Can you work these out from the model? Positions are in its coordinate system, mm. Face numbers are marked on the shaded views. A direction names the side the tool comes from. Round coordinates to 2 decimals unless told otherwise and drop trailing zeros. Loops run counter-clockwise (first coordinate to the right, second up) from the corner with the lowest first, then second, coordinate; pieces in that order, holes last. Notation, with made-up numbers: (1, 40.5) - (58, 40.5) arc R21 cw to (58, 59.5) - close; hole circle Ø4 at (4.5, 21). An arc over 180 degrees is marked (long way). Answer as CSV lines item,"result".
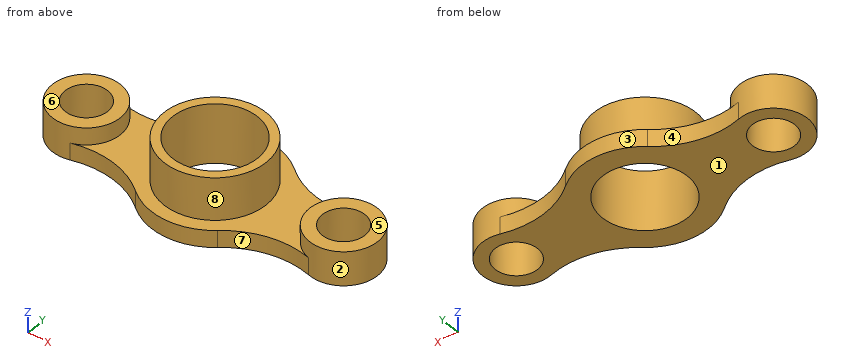
```python
from build123d import *

# Parameters (mm, degrees)
SKETCH2_R           = 60
BOSS_EXTRUDE1_DEPTH = 20
SKETCH2_5_R         = 40
SKETCH2_5_R_2       = 25
BOSS_EXTRUDE4_DEPTH = 40
SKETCH2_6_R         = 60
SKETCH2_6_R_2       = 50
BOSS_EXTRUDE5_DEPTH = 70


with BuildPart() as part:
    # Sketch2 → Boss-Extrude1 (new body)
    with BuildSketch(Plane.XY):
        with BuildLine():
            ThreePointArc((-139.071428571, -38.478127898), (-91.104177178, -36.827906099), (-47.892857143, -57.717191847))
            ThreePointArc((-47.892857143, -57.717191847), (0, -75), (47.892857143, -57.717191847))
            ThreePointArc((47.892857143, -57.717191847), (91.104177178, -36.827906099), (139.071428571, -38.478127898))
            ThreePointArc((139.071428571, -38.478127898), (110, 0), (139.071428571, 38.478127898))
            ThreePointArc((139.071428571, 38.478127898), (91.104177178, 36.827906099), (47.892857143, 57.717191847))
            ThreePointArc((47.892857143, 57.717191847), (0, 75), (-47.892857143, 57.717191847))
            ThreePointArc((-47.892857143, 57.717191847), (-91.104177178, 36.827906099), (-139.071428571, 38.478127898))
            ThreePointArc((-139.071428571, 38.478127898), (-118.084934144, 24.112830017), (-110, 0))
            ThreePointArc((-110, 0), (-118.084934144, -24.112830017), (-139.071428571, -38.478127898))
        make_face()
        Circle(SKETCH2_R, mode=Mode.SUBTRACT)
    extrude(amount=BOSS_EXTRUDE1_DEPTH)

    # Sketch2_5 → Boss-Extrude4 (add)
    # profile 1 of 2: a face of its own
    with BuildSketch(Plane.XY):
        with Locations(Location((-150, 0, 0), (0, 0, 74.144374523))):
            Circle(SKETCH2_5_R)
        with Locations((-150, 0)):
            Circle(SKETCH2_5_R_2, mode=Mode.SUBTRACT)
    # profile 2 of 2: a face of its own
    with BuildSketch(Plane.XY):
        with Locations(Location((150, 0, 0), (0, 0, 105.855625477))):
            Circle(SKETCH2_5_R)
        with Locations((150, 0)):
            Circle(SKETCH2_5_R_2, mode=Mode.SUBTRACT)
    extrude(amount=BOSS_EXTRUDE4_DEPTH)

    # Sketch2_6 → Boss-Extrude5 (add)
    with BuildSketch(Plane.XY):
        Circle(SKETCH2_6_R)
        Circle(SKETCH2_6_R_2, mode=Mode.SUBTRACT)
    extrude(amount=BOSS_EXTRUDE5_DEPTH)


solid = part.part
```
Q1. Imagine slicing it at A-A (x = -150). Write out the boundary of the cut face in (y, z).
Checks:
outline,"(-40, 0) - (-25, 0) - (-25, 40) - (-40, 40) - close; (25, 0) - (40, 0) - (40, 40) - (25, 40) - close"
Q2. We'd pull the mould along X, two halves only. Please class the marked faces 1, 2 and 3: pulls with the +X half, pulls with the -X half, needs draft (parallel to the pull), parting line crosses it, or undercut.
Checks:
face 1,"needs draft"
face 2,"undercut"
face 3,"parting line crosses it"
Q3. On a 3-axis mill with a long thin cutter (end or side, diameter ignored), from which of +Z, -Z, +X, -X, +Y, -Y can I reach the whole of each face in a straight line? I mean the marked faces 4, 5, 6, 7 and 8. Say none if no direction works.
Checks:
face 4,"+Z, -Z, +Y"
face 5,"+Z, +X, +Y, -Y"
face 6,"+Z, -X, +Y, -Y"
face 7,"+Z, -Z, -Y"
face 8,"+Z"
Q4. I'm going to push flat-ended pins straight in: pin 1 Ø4 at (x, z) = (73.5, 11.5) entering from -Y; pin 2 Ø4 at (y, z) = (25.5, 19.5) entering from +X; pin 3 Ø3 at (x, y) = (76, 26) entering from +Z. Where does each tip first touch, or does it pass through?
Checks:
pin 1,"y = -43.13"
pin 2,"x = 182.37"
pin 3,"z = 20"
Q5. Imagine slicing it at D-D (x = 0). Write out the boundary of the cut face in (y, z).
Checks:
outline,"(-75, 0) - (-50, 0) - (-50, 70) - (-60, 70) - (-60, 20) - (-75, 20) - close; (50, 0) - (75, 0) - (75, 20) - (60, 20) - (60, 70) - (50, 70) - close"
Q6. Imagine slicing it at C-C (z = 16). Write out the boundary of the cut face in (x, y).
Checks:
outline,"(-139.07, -38.48) arc R100 cw to (-47.89, -57.72) arc R75 ccw to (47.89, -57.72) arc R100 cw to (139.07, -38.48) arc R40 ccw (long way) to (139.07, 38.48) arc R100 cw to (47.89, 57.72) arc R75 ccw to (-47.89, 57.72) arc R100 cw to (-139.07, 38.48) arc R40 ccw (long way) to start; hole circle Ø50 at (-150, 0); hole circle Ø100 at (0, 0); hole circle Ø50 at (150, 0)"
Q7. If I drill on line 1 along Y through (x, z) = (150, 13.5); line 2 along X through (y, z) = (21, 11); line 3 along Z through (x, y) = (-50.5, 54.5), over which ranges is the centre line in solid material (lowest first)? Write a range as [from, to].
Checks:
line 1,"[-40, -25], [25, 40]"
line 2,"[-184.04, -163.56], [-136.44, -45.38], [45.38, 136.44], [163.56, 184.04]"
line 3,"[0, 20]"
Q8. Imagine slicing it at B-B (y = 0). Write out the boundary of the cut face in (x, z), then the cut area to 3 significant figures.
Checks:
outline,"(-190, 0) - (-175, 0) - (-175, 40) - (-190, 40) - close; (-125, 0) - (-50, 0) - (-50, 70) - (-60, 70) - (-60, 20) - (-110, 20) - (-110, 40) - (-125, 40) - close; (50, 0) - (125, 0) - (125, 40) - (110, 40) - (110, 20) - (60, 20) - (60, 70) - (50, 70) - close; (175, 0) - (190, 0) - (190, 40) - (175, 40) - close"
area,"5,800 mm²"
